Verification items for the finished model (mm, model axes). Round coordinates to 2 decimals unless told otherwise and drop trailing zeros. Write each loop counter-clockwise with the first axis right and the second up, starting at its lowest first coordinate (ties: lowest second). Pieces come first, ordered by that corner, then holes. Notation, with made-up numbers: M 16.5,-22.5 L 27.5,-22.5 A25 cw 27.5,10.5 Z; hole C 58,57.5 d9. An arc over 180 degrees is marked long. One line per item, written item: value. Start each with the question number.
Item 1: Gauge pin test, flat end, axial feed: pin 1 (2 mm diameter, centred on x = 16.5, y = -28.5, fed in from +Z). Record the tip position at first contact, or that the pin passes through.
Item 2: Draft check along Y on faces 1 (the face through (22, -39.267, 13)), 2 (the face through (22, -29, 1)), 3 (the face through (22, -58, 24.8)). Enter one of: +Y half, -Y half, draft (parallel to the pull), parting line (faces both ways), or undercut.
Item 3: Section check A-A, the plane y = -107. Record the cut outline in (x, z), then the cut area to 3 significant figures.
Item 4: Thickness scan on probe 1 along X at (y, z) = (-61.5, 16.25); probe 2 along Z at (x, y) = (25, -88). Record the ranges inside material, lowest first. Write a range as from..to.
Item 5: Section check B-B, the plane z = 14.5. State how many separate pieces and enclosed holes the cut face has, then the cut area to 3 significant figures.
from build123d import *

# Parameters (mm, degrees)
F0_W     = 43.8
F0_H     = 115.8
F1_DEPTH = 24.8
F2_W     = 41.8
F2_H     = 18.133333
F2_H_2   = 18.133334
F3_DEPTH = 23.8
F4_R     = 0.5
F5_R     = 0.5
F6_R     = 0.5


with BuildPart() as f1:
    # F0 (on Top) → F1 (new body)
    with BuildSketch(Plane.XY):
        with Locations((21.9, -57.9)):
            Rectangle(F0_W, F0_H)
    extrude(amount=F1_DEPTH)

    # F2 (on face) → F3 (cut)
    with BuildSketch(Plane.XY.offset(24.8)):
        with Locations((21.9, -10.066667)):
            Rectangle(F2_W, F2_H)
        with Locations((21.9, -29.2)):
            Rectangle(F2_W, F2_H_2)
        with Locations((21.9, -48.333333)):
            Rectangle(F2_W, F2_H)
        with Locations((21.9, -67.466667)):
            Rectangle(F2_W, F2_H)
        with Locations((21.9, -86.6)):
            Rectangle(F2_W, F2_H_2)
        with Locations((21.9, -105.733333)):
            Rectangle(F2_W, F2_H)
    extrude(amount=-F3_DEPTH, mode=Mode.SUBTRACT)

    # F4
    f4_edges = [f1.edges().sort_by_distance(p)[0] for p in [
        (43.8, 0, 12.4),
        (43.8, -115.8, 12.4),
        (0, -115.8, 12.4),
        (0, 0, 12.4),
        (0, -57.9, 0),
        (21.9, -115.8, 0),
        (21.9, 0, 0),
        (43.8, -57.9, 0),
    ]]
    fillet(f4_edges, radius=F4_R)

    # F5
    f5_edges = [f1.edges().sort_by_distance(p)[0] for p in [
        (1, -1, 12.9),
        (42.8, -1, 12.9),
        (42.8, -20.133333, 12.9),
        (42.8, -39.266667, 12.9),
        (42.8, -58.4, 12.9),
        (42.8, -77.533333, 12.9),
        (42.8, -96.666667, 12.9),
        (42.8, -114.8, 12.9),
        (1, -114.8, 12.9),
        (1, -95.666667, 12.9),
        (1, -76.533333, 12.9),
        (1, -57.4, 12.9),
        (1, -38.266667, 12.9),
        (1, -19.133333, 12.9),
    ]]
    fillet(f5_edges, radius=F5_R)

    # F6
    f6_edges = [f1.edges().sort_by_distance(p)[0] for p in [
        (42.8, -19.133333, 12.9),
        (42.8, -38.266667, 12.9),
        (42.8, -57.4, 12.9),
        (1, -20.133333, 12.9),
        (1, -39.266667, 12.9),
        (1, -58.4, 12.9),
        (42.8, -76.533333, 12.9),
        (42.8, -95.666667, 12.9),
        (1, -77.533333, 12.9),
        (1, -96.666667, 12.9),
    ]]
    fillet(f6_edges, radius=F6_R)


solid = f1.part
Response values:
1. pin 1: stops at z = 1
2. face 1: undercut
2. face 2: undercut
2. face 3: draft
3. outline: M 0,0.5 A0.5 ccw 0.5,0 L 43.3,0 A0.5 ccw 43.8,0.5 L 43.8,24.8 L 42.8,24.8 L 42.8,1 L 1,1 L 1,24.8 L 0,24.8 Z
3. area: 91.3 mm2
4. probe 1: x = 0..1, 42.8..43.8
4. probe 2: z = 0..1
5. separate pieces: 1
5. enclosed holes: 6
5. area: 525 mm2
